Model file for the job. Use its own axes, mm. A direction names the side the tool comes from. Coordinates: 2 decimals unless noted, no trailing zeros. Write each loop counter-clockwise with the first axis right and the second up, starting at its lowest first coordinate (ties: lowest second). Pieces come first, ordered by that corner, then holes.
Q1. Band-saw the part on A-A, the plane z = 0. Write the cut outline in (x, y).
Q2. Band-saw the part on B-B, the plane y = -14. Write the cut outline in (x, z), plus the area to 3 significant figures.
Q3. Pull direction X, two halves, no side cores. Call faces 5 (the flat face through (3, -16, -3)), 6 (the cylindrical face through (-2.699, -26.253, -7.615)), 7 (the flat face through (-2, 0, 0)), 8 (the flat face through (0, -14.45, 0)): released by +X, released by -X, zero draft, split by the parting line, or undercut.
Q4. Pin check, flat tips, straight feed: P1, Ø8, axis at x = -13, z = -2.5, coming from the +Y side; P2, Ø1, axis at x = -3, y = -22.5, coming from the -Z side; P3, Ø2.5, axis at x = -29, y = -25.35, coming from the +Z side; P4, Ø0.9, axis at x = 0.5, z = 0, coming from the +Y side. Stop position of each tip, or through.
Q5. Which spindle directions (+Z, -Z, +X, -X, +Y, -Y) get a long thin tool onto all of the face, cutting with end or side? Do faces 1 (the flat face through (0, -16, -2.1)), 2 (the flat face through (-5, -9, -7)), 3 (the flat face through (-26, -26, 1)), 4 (the flat face through (-26, -9, 0)). Say none if no direction does.
Q6. Band-saw the part on D-D, the plane y = -21.5. Write the cut outline in (x, z).
Q7. Drill centre lines: probe 1 along X at (y, z) = (-4, 0); probe 2 along Y at (x, z) = (0, 2.75); probe 3 along X at (y, z) = (-29, -2). Where is each one in solid material? Low to high.
Q8. Band-saw the part on C-C, the plane x = 0. Write the cut outline in (y, z), plus the area to 3 significant figures.
from build123d import *

# Parameters (mm, degrees)
SKETCH1_R           = 1.5
BOSS_EXTRUDE1_DEPTH = 19.45
BOSS_EXTRUDE2_START = -5
SKETCH2_R           = 1.5
BOSS_EXTRUDE2_DEPTH = 5
SKETCH5_W           = 35
SKETCH5_H           = 15.8
BOSS_EXTRUDE3_DEPTH = 2
SKETCH6_R           = 1.5
BOSS_EXTRUDE4_DEPTH = 15.8
SKETCH7_W           = 19
SKETCH7_H           = 2
BOSS_EXTRUDE5_DEPTH = 15.8
SKETCH8_W           = 8
SKETCH8_H           = 2
CUT_EXTRUDE1_DEPTH  = 10
FILLET1_R           = 1
SKETCH9_W           = 23
SKETCH9_H           = 2
CUT_EXTRUDE2_DEPTH  = 44
FILLET2_R           = 1


with BuildPart() as part:
    # Sketch1 → Boss-Extrude1 (new body)
    with BuildSketch(Plane(origin=(0, 0, 0), x_dir=(1, 0, 0), z_dir=(0, 1, 0))):
        Polygon((-5, 7.9), (3, 7.9), (3, 5.9), (3, -5.9), (3, -7.9), (-5, -7.9), (-5, -5.9), (-3, -5.9), (-3, 5.9), (-5, 5.9), align=None)
        with Locations(Location((0, 0, 0), (0, 0, 270))):
            Circle(SKETCH1_R, mode=Mode.SUBTRACT)
    extrude(amount=-BOSS_EXTRUDE1_DEPTH)

    # Sketch2 → Boss-Extrude2 (add)
    with BuildSketch(Plane.XZ.offset(19.45).offset(BOSS_EXTRUDE2_START)):
        with Locations(Location((0, 0, 0), (0, 0, 90))):
            Circle(SKETCH2_R)
    extrude(amount=BOSS_EXTRUDE2_DEPTH)


with BuildPart() as body_2:
    # Mirror2: mirrored copy
    add(part.part.mirror(Plane.ZY.offset(14.5)))


with BuildPart() as part_1:
    add(part.part)

    add(body_2.part)  # Boss-Extrude3 merges body 2
    # Sketch5 → Boss-Extrude3 (add)
    with BuildSketch(Plane.XZ.offset(19.45)):
        with Locations((-14.5, 0)):
            Rectangle(SKETCH5_W, SKETCH5_H)
    extrude(amount=-BOSS_EXTRUDE3_DEPTH)

    # Sketch6 → Boss-Extrude4 (add)
    # profile 1 of 2: a face of its own
    with BuildSketch(Plane.XY.offset(7.9)):
        Polygon((-26, -31.25), (-26, -19.45), (-32, -19.45), (-32, -31.25), (-32, -33.25), (-24, -33.25), (-24, -31.25), align=None)
        with Locations((-29, -25.35)):
            Circle(SKETCH6_R, mode=Mode.SUBTRACT)
    # profile 2 of 2: a face of its own
    with BuildSketch(Plane.XY.offset(7.9)):
        Polygon((-3, -19.45), (-3, -31.25), (-5, -31.25), (-5, -33.25), (3, -33.25), (3, -31.25), (3, -19.45), align=None)
        with Locations((0, -25.35)):
            Circle(SKETCH6_R, mode=Mode.SUBTRACT)
    extrude(amount=-BOSS_EXTRUDE4_DEPTH)

    # Sketch7 → Boss-Extrude5 (add)
    with BuildSketch(Plane.XY.offset(7.9)):
        with Locations((-14.5, -32.25)):
            Rectangle(SKETCH7_W, SKETCH7_H)
    extrude(amount=-BOSS_EXTRUDE5_DEPTH)

    # Sketch8 → Cut-Extrude1 (cut)
    with BuildSketch(Plane.XY.offset(7.9)):
        with Locations((-1, -16.45)):
            Rectangle(SKETCH8_W, SKETCH8_H)
    extrude(amount=-CUT_EXTRUDE1_DEPTH, mode=Mode.SUBTRACT)

    # Fillet1
    fillet1_edges = [part_1.edges().sort_by_distance(p)[0] for p in [
        (3, -15.45, 2.9),
        (-1, -15.45, 7.9),
    ]]
    fillet(fillet1_edges, radius=FILLET1_R)

    # Sketch9 → Cut-Extrude2 (cut)
    with BuildSketch(Plane.XY.offset(7.9)):
        with Locations((-14.5, -32.25)):
            Rectangle(SKETCH9_W, SKETCH9_H)
    extrude(amount=-CUT_EXTRUDE2_DEPTH, mode=Mode.SUBTRACT)

    # Fillet2
    fillet2_edges = [part_1.edges().sort_by_distance(p)[0] for p in [
        (-26, -26.35, -7.9),
        (-3, -26.35, -7.9),
    ]]
    fillet(fillet2_edges, radius=FILLET2_R)


solid = part_1.part
Answer sheet:
1. outline: (-32, -33.25) - (-26, -33.25) - (-26, -19.45) - (-3, -19.45) - (-3, -33.25) - (3, -33.25) - (3, -17.45) - (-26, -17.45) - (-26, 0) - (-27.5, 0) - (-27.5, -14.45) - (-30.5, -14.45) - (-30.5, 0) - (-32, 0) - close; (-3, -15.45) - (2, -15.45) arc R1 ccw to (3, -14.45) - (3, 0) - (1.5, 0) - (1.5, -14.45) - (-1.5, -14.45) - (-1.5, 0) - (-3, 0) - close; hole circle Ø3 at (-29, -25.35); hole circle Ø3 at (0, -25.35)
2. outline: (-32, -7.9) - (-24, -7.9) - (-24, -5.9) - (-26, -5.9) - (-26, 5.9) - (-24, 5.9) - (-24, 7.9) - (-32, 7.9) - close; (-5, -7.9) - (3, -7.9) - (3, 7.9) - (-5, 7.9) - (-5, 5.9) - (-3, 5.9) - (-3, -5.9) - (-5, -5.9) - close; hole circle Ø3 at (-29, 0); hole circle Ø3 at (0, 0)
2. area: 191 mm2
3. face 5: released by +X
3. face 6: undercut
3. face 7: zero draft
3. face 8: undercut
4. P1: stops at y = -17.45
4. P2: stops at z = -7.77
4. P3: passes through
4. P4: stops at y = -14.45
5. face 1: +Z, +X
5. face 2: +Z, -Z, +Y
5. face 3: +Z, -Z, -Y
5. face 4: +Y
6. outline: (-32, -7.9) - (-27, -7.9) arc R1 ccw to (-26, -6.9) - (-26, 7.9) - (-32, 7.9) - close; (-3, -6.9) arc R1 ccw to (-2, -7.9) - (3, -7.9) - (3, 7.9) - (-3, 7.9) - close
7. probe 1: x = -32 to -30.5, -27.5 to -26, -3 to -1.5, 1.5 to 3
7. probe 2: y = -33.25 to -26.85, -23.85 to -17.45, -15.45 to 0
7. probe 3: x = -32 to -26, -3 to 3
8. outline: (-33.25, -7.9) - (-26.85, -7.9) - (-26.85, 7.9) - (-33.25, 7.9) - close; (-23.85, -7.9) - (0, -7.9) - (0, -1.5) - (-14.45, -1.5) - (-14.45, 1.5) - (0, 1.5) - (0, 7.9) - (-14.45, 7.9) arc R1 ccw to (-15.45, 6.9) - (-15.45, -2.1) - (-17.45, -2.1) - (-17.45, 7.9) - (-23.85, 7.9) - close
8. area: 414 mm2
